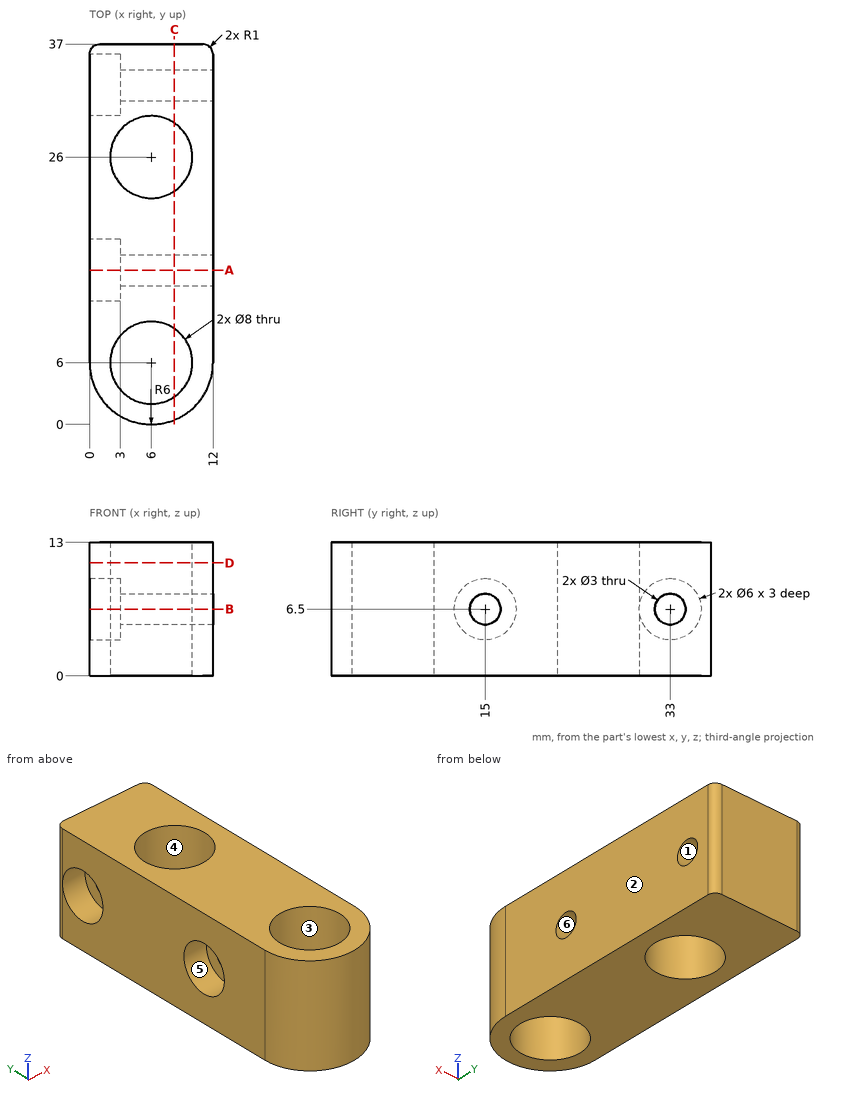
Verification items for this drawing (mm, ordinates from the low corner). A direction names the side the tool comes from. Coordinates: 2 decimals unless noted, no trailing zeros. Write each loop counter-clockwise with the first axis right and the second up, starting at its lowest first coordinate (ties: lowest second). Pieces come first, ordered by that corner, then holes. Notation, with made-up numbers: (1.5, 79.5) -> (18.5, 79.5) arc R30 ccw to (18.5, 118.5) -> close; hole circle Ø7 at (72, -34.75). An arc over 180 degrees is marked (long way). One line per item, written item: value. Start each with the question number.
Q1. Cross-section at D-D on z = 11. Enter the section's corners in (x, y).
Q2. Go/stop test with flat-tipped pins: P1, Ø1.8, axis at y = 15, z = 6.5, coming from the +X side; P2, Ø5, axis at y = 33, z = 6.5, coming from the -X side. Record where each tip stops, or that it passes through.
Q3. Thickness scan on L1, parallel to Z at x = 9.5, y = 33; L2, parallel to Y at x = 6, z = 4; L3, parallel to Y at x = 7.5, z = 10.5. Record the ranges inside material, lowest first. Write a range as from..to.
Q4. Mould release check, pull along X, two halves, no side actions. Record for the marked faces 1, 2, 3 and 4: pulls with the +X half, pulls with the -X half, needs draft (parallel to the pull), parting line crosses it, or undercut.
Q5. Cross-section at B-B on z = 6.5. State how many separate pieces and enclosed holes the cut face has.
Q6. Cross-section at A-A on y = 15. Enter the section's corners in (x, z), and give its area (3 significant figures).
Q7. Access from +Z, -Z, +X, -X, +Y, -Y to the whole of each face (thin tool, end or side, straight path). Record for the marked faces 5 and 6.
Q8. Cross-section at C-C on x = 8.25. Enter the section's corners in (y, z).
Checked values:
1. outline: (0, 6) arc R6 ccw to (12, 6) -> (12, 36) arc R1 ccw to (11, 37) -> (1, 37) arc R1 ccw to (0, 36) -> close; hole circle Ø8 at (6, 6); hole circle Ø8 at (6, 26)
2. P1: passes through
2. P2: stops at x = 3
3. L1: z = 0..5, 8..13
3. L2: y = 0..2, 10..22, 30..37
3. L3: y = 0.19..2.29, 9.71..22.29, 29.71..37
4. face 1: needs draft
4. face 2: pulls with the +X half
4. face 3: undercut
4. face 4: undercut
5. separate pieces: 3
5. enclosed holes: 2
6. outline: (0, 0) -> (12, 0) -> (12, 5) -> (3, 5) -> (3, 3.5) -> (0, 3.5) -> close; (0, 9.5) -> (3, 9.5) -> (3, 8) -> (12, 8) -> (12, 13) -> (0, 13) -> close
6. area: 111 mm²
7. face 5: -X
7. face 6: +X, -X
8. outline: (0.44, 0) -> (2.69, 0) -> (2.69, 13) -> (0.44, 13) -> close; (9.31, 0) -> (22.69, 0) -> (22.69, 13) -> (9.31, 13) -> close; (29.31, 0) -> (37, 0) -> (37, 13) -> (29.31, 13) -> close; hole circle Ø3 at (15, 6.5); hole circle Ø3 at (33, 6.5)
